from build123d import *

# Parameters (mm, degrees)
SKETCH1_R           = 4
SKETCH1_R_2         = 3.5
SKETCH1_R_3         = 2.5
BOSS_EXTRUDE1_DEPTH = 10
SKETCH2_W           = 25
SKETCH2_H           = 1
CUT_EXTRUDE1_DEPTH  = 10


with BuildPart() as part:
    # Sketch1 → Boss-Extrude1 (new body)
    with BuildSketch(Plane.XY):
        with BuildLine():
            Line((40, 67), (50, 57))
            Line((50, 57), (50, 0))
            Line((50, 0), (5, 0))
            ThreePointArc((5, 0), (1.464466094, 1.464466094), (0, 5))
            Line((0, 5), (0, 62))
            ThreePointArc((0, 62), (1.464466094, 65.535533906), (5, 67))
            Line((5, 67), (40, 67))
        make_face()
        with Locations((10, 57)):
            Circle(SKETCH1_R, mode=Mode.SUBTRACT)
        with Locations((25, 57)):
            Circle(SKETCH1_R_2, mode=Mode.SUBTRACT)
        with Locations((40, 57)):
            Circle(SKETCH1_R_3, mode=Mode.SUBTRACT)
        with Locations((10, 42)):
            Circle(SKETCH1_R, mode=Mode.SUBTRACT)
        with Locations((25, 42)):
            Circle(SKETCH1_R_2, mode=Mode.SUBTRACT)
        with Locations((40, 42)):
            Circle(SKETCH1_R_3, mode=Mode.SUBTRACT)
    extrude(amount=BOSS_EXTRUDE1_DEPTH)

    # Sketch2 → Cut-Extrude1 (cut)
    with BuildSketch(Plane.XY.offset(10)):
        with Locations((37.5, 25.5)):
            Rectangle(SKETCH2_W, SKETCH2_H)
        with Locations((37.5, 16.5)):
            Rectangle(SKETCH2_W, SKETCH2_H)
        with Locations((37.5, 7.5)):
            Rectangle(SKETCH2_W, SKETCH2_H)
    extrude(amount=-CUT_EXTRUDE1_DEPTH, mode=Mode.SUBTRACT)


solid = part.part
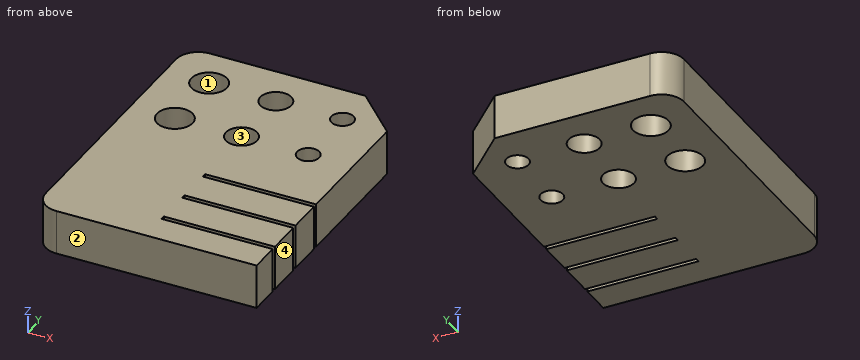
Read the model definition and answer for the solid it produces. Units are mm, in the model's axes. Face numbers are marked on the shaded views. Round coordinates to 2 decimals unless told otherwise and drop trailing zeros. Write each loop counter-clockwise with the first axis right and the second up, starting at its lowest first coordinate (ties: lowest second). Pieces come first, ordered by that corner, then holes.
Q1. Find section C-C on z = 7. Determine the outline of the cut face in (x, y), and give its area (3 significant figures).
Values:
outline: (0, 5) arc R5 ccw to (5, 0) - (50, 0) - (50, 7) - (25, 7) - (25, 8) - (50, 8) - (50, 16) - (25, 16) - (25, 17) - (50, 17) - (50, 25) - (25, 25) - (25, 26) - (50, 26) - (50, 57) - (40, 67) - (5, 67) arc R5 ccw to (0, 62) - close; hole circle Ø8 at (10, 42); hole circle Ø8 at (10, 57); hole circle Ø7 at (25, 42); hole circle Ø7 at (25, 57); hole circle Ø5 at (40, 42); hole circle Ø5 at (40, 57)
area: 3,000 mm2
Q2. Find section B-B on y = 42. Determine the outline of the cut face in (x, z), and give its area (3 significant figures).
Values:
outline: (0, 0) - (6, 0) - (6, 10) - (0, 10) - close; (14, 0) - (21.5, 0) - (21.5, 10) - (14, 10) - close; (28.5, 0) - (37.5, 0) - (37.5, 10) - (28.5, 10) - close; (42.5, 0) - (50, 0) - (50, 10) - (42.5, 10) - close
area: 300 mm2
Q3. The mould has two halves that part along Y. Classify the marked faces 1, 2, 3 and 4: released by +Y, released by -Y, zero draft, split by the parting line, or undercut.
Values:
face 1: undercut
face 2: released by -Y
face 3: undercut
face 4: zero draft
Q4. Straight lines are drawn through the part: line 1 (Y direction, x = 40, z = 3.5); line 2 (Y direction, x = 46.5, z = 0.75); line 3 (Y direction, x = 31.5, z = 8.25). For each, find the intervals that lie inside material, in ascending order.
Values:
line 1: y = 0 to 7, 8 to 16, 17 to 25, 26 to 39.5, 44.5 to 54.5, 59.5 to 67
line 2: y = 0 to 7, 8 to 16, 17 to 25, 26 to 60.5
line 3: y = 0 to 7, 8 to 16, 17 to 25, 26 to 67
Q5. Flat-ended cylindrical pins translate along their axes: P1, Ø5, axis at x = 43, z = 3, coming from the +Y side; P2, Ø5, axis at x = 43.5, z = 3, coming from the +Y side; P3, Ø4.5, axis at x = 40, y = 42, coming from the +Z side. Find the tip coordinate at first contact, or state that the pin passes through.
Values:
P1: stops at y = 66.5
P2: stops at y = 66
P3: passes through
Q6. Find section D-D on x = 27.5. Determine the outline of the cut face in (y, z), and give its area (3 significant figures).
Values:
outline: (0, 0) - (7, 0) - (7, 10) - (0, 10) - close; (8, 0) - (16, 0) - (16, 10) - (8, 10) - close; (17, 0) - (25, 0) - (25, 10) - (17, 10) - close; (26, 0) - (39.55, 0) - (39.55, 10) - (26, 10) - close; (44.45, 0) - (54.55, 0) - (54.55, 10) - (44.45, 10) - close; (59.45, 0) - (67, 0) - (67, 10) - (59.45, 10) - close
area: 542 mm2
Q7. Find section A-A on x = 10. Determine the outline of the cut face in (y, z).
Values:
outline: (0, 0) - (38, 0) - (38, 10) - (0, 10) - close; (46, 0) - (53, 0) - (53, 10) - (46, 10) - close; (61, 0) - (67, 0) - (67, 10) - (61, 10) - close
